Read the model definition and answer for the solid it produces. Units are mm, in the model's axes. A direction names the side the tool comes from. Coordinates: 2 decimals unless noted, no trailing zeros. Order: outer loops, then holes, each group sorted by start corner. A loop starts at its lowest first (then second) coordinate and runs counter-clockwise, first axis right, second up. Notation, with made-up numbers: (3, 26.5) - (48, 26.5) arc R23 ccw to (48, 44.5) - close; hole circle Ø7 at (-39.5, 20.25). An arc over 180 degrees is marked (long way). Use one line per item in the form item = value.
```python
from build123d import *

# Parameters (mm, degrees)
BOSS_EXTRUDE1_OUTLINE_R = 1.75
BOSS_EXTRUDE1_DEPTH     = 4
CUT_EXTRUDE1_DEPTH      = 1


# Read off the part's stored shape, not the designer's step: Boss-Extrude1
with BuildPart() as part:
    # Boss-Extrude1 outline → Boss-Extrude1 (new body)
    with BuildSketch(Plane(origin=(0, 0, 0), x_dir=(1, 0, 0), z_dir=(0, 1, 0))):
        with BuildLine():
            Line((24.866474615, -10.33744254), (35.59307775, -10.33744254))
            ThreePointArc((35.59307775, -10.33744254), (38.029776183, -5.587442326), (40.466474615, -10.33744254))
            Line((40.466474615, -10.33744254), (47.529776182, -10.33744254))
            Line((47.529776182, -10.33744254), (47.529776182, -18.81631662))
            Line((47.529776182, -18.81631662), (58.529776182, -18.81631662))
            Line((58.529776182, -18.81631662), (58.529776182, -4.977921711))
            Line((58.529776182, -4.977921711), (-21.470223818, -4.977921711))
            Line((-21.470223818, -4.977921711), (-21.470223818, -18.81631662))
            Line((-21.470223818, -18.81631662), (-10.470223818, -18.81631662))
            Line((-10.470223818, -18.81631662), (-10.470223818, -10.33744254))
            Line((-10.470223818, -10.33744254), (4.39307775, -10.33744254))
            ThreePointArc((4.39307775, -10.33744254), (6.829776182, -5.587442326), (9.266474615, -10.33744254))
            Line((9.266474615, -10.33744254), (19.99307775, -10.33744254))
            ThreePointArc((19.99307775, -10.33744254), (22.429776182, -5.587442326), (24.866474615, -10.33744254))
        make_face()
        with Locations((-16.470223818, -13.587442433)):
            Circle(BOSS_EXTRUDE1_OUTLINE_R, mode=Mode.SUBTRACT)
        with Locations((53.529776182, -13.587442433)):
            Circle(BOSS_EXTRUDE1_OUTLINE_R, mode=Mode.SUBTRACT)
    extrude(amount=BOSS_EXTRUDE1_DEPTH)

    # Sketch2 → Cut-Extrude1 (cut)
    # profile 1 of 2: a face of its own
    with BuildSketch(Plane(origin=(0, 4, 0), x_dir=(1, 0, 0), z_dir=(0, 1, 0))):
        Polygon((-16.41198232, -6.812466594), (-14.865187448, -6.812466594), (-14.865187448, -7.382338389), (-15.842110525, -7.382338389), (-15.842110525, -7.992915312), (-14.865187448, -7.992915312), (-14.865187448, -8.562787107), (-15.842110525, -8.562787107), (-15.842110525, -9.987466594), (-16.41198232, -9.987466594), align=None)
    # profile 2 of 2: a face of its own
    with BuildSketch(Plane(origin=(0, 4, 0), x_dir=(1, 0, 0), z_dir=(0, 1, 0))):
        Polygon((-13.260514973, -6.731056337), (-12.667110525, -6.731056337), (-12.667110525, -8.807017876), (-12.382174628, -8.807017876), (-12.382174628, -9.336184543), (-12.667110525, -9.336184543), (-12.667110525, -9.987466594), (-13.23698232, -9.987466594), (-13.23698232, -9.336184543), (-14.580251551, -9.336184543), (-14.580251551, -8.759316554), align=None)
        Polygon((-13.23698232, -8.807017876), (-13.23698232, -7.726423926), (-13.939781799, -8.807017876), align=None, mode=Mode.SUBTRACT)
    extrude(amount=-CUT_EXTRUDE1_DEPTH, mode=Mode.SUBTRACT)


solid = part.part
```
(1) Which of the six approach directions +Z, -Z, +X, -X, +Y, -Y give full straight-line access (tool end or side, diameter ignored) to faces 1 (the cylindrical face through (37.94, 1.97, 5.59)), 2 (the flat face through (44, 2, 10.337))?
Answer list:
face_1 = +Y, -Y
face_2 = +Z, +Y, -Y
(2) Section C-C, the plane x = 3 is taken. Write down the section's boundary in (y, z).
Answer list:
outline = (0, 4.98) - (4, 4.98) - (4, 10.34) - (0, 10.34) - close
(3) Given pin 1 Ø1.2 at (x, z) = (-15.5, 8.5) entering from +Y; pin 2 Ø1.2 at (x, y) = (16.5, 2) entering from +Z, each flat-ended and moving along its own axis, determine where each tip first touches the part or whether it passes through.
Answer list:
pin_1 = 4
pin_2 = 10.34
(4) The mould has two halves that part along Z. Classify faces 3 (the flat face through (19, 2, 4.978)), 4 (the flat face through (-13.93, 3.51, 7.76)), 5 (the flat face through (-3, 2, 10.337)): +Z half, -Z half, draft (parallel to the pull), parting line (faces both ways), or undercut.
Answer list:
face_3 = -Z half
face_4 = undercut
face_5 = +Z half
(5) Straight lines are drawn through the part: L1, parallel to X at y = 1.05, z = 8.75; L2, parallel to X at y = 3.5, z = 17; L3, parallel to X at y = 1.25, z = 8. For each, find the intervals that lie inside material, in ascending order.
Answer list:
L1 = -21.47 to 3.83, 9.83 to 19.43, 25.43 to 35.03, 41.03 to 58.53
L2 = -21.47 to -10.47, 47.53 to 58.53
L3 = -21.47 to 3.89, 9.77 to 19.49, 25.37 to 35.09, 40.97 to 58.53
(6) Section B-B, the plane z = 14.5 is taken. Write down the section's boundary in (x, y), then the cut area to 3 significant figures.
Answer list:
outline = (-21.47, 0) - (-17.96, 0) - (-17.96, 4) - (-21.47, 4) - close; (-14.98, 0) - (-10.47, 0) - (-10.47, 4) - (-14.98, 4) - close; (47.53, 0) - (52.04, 0) - (52.04, 4) - (47.53, 4) - close; (55.02, 0) - (58.53, 0) - (58.53, 4) - (55.02, 4) - close
area = 64.1 mm2
(7) Section A-A, the plane y = 1.7 is taken. Write down the section's boundary in (x, z).
Answer list:
outline = (-21.47, 4.98) - (58.53, 4.98) - (58.53, 18.82) - (47.53, 18.82) - (47.53, 10.34) - (40.47, 10.34) arc R3 cw (long way) to (35.59, 10.34) - (24.87, 10.34) arc R3 cw (long way) to (19.99, 10.34) - (9.27, 10.34) arc R3 cw (long way) to (4.39, 10.34) - (-10.47, 10.34) - (-10.47, 18.82) - (-21.47, 18.82) - close; hole circle Ø3.5 at (-16.47, 13.59); hole circle Ø3.5 at (53.53, 13.59)
